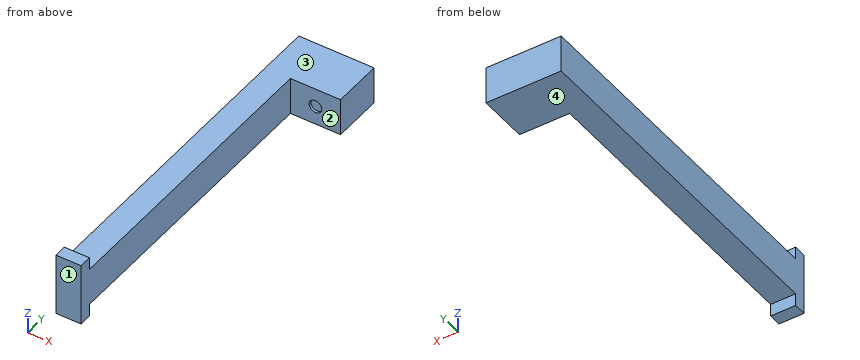
```python
from build123d import *

# Parameters (mm, degrees)
SKETCH2_W                = 30
SKETCH2_H                = 20
SKETCH2_W_2              = 10
SKETCH2_H_2              = 120
BOSS_EXTRUDE1_DEPTH      = 15
SKETCH3_W                = 10
SKETCH3_H                = 5
BOSS_EXTRUDE2_DEPTH      = 5
BOSS_EXTRUDE2_DEPTH_BACK = 20
SKETCH5_R                = 2.517277228
CUT_EXTRUDE1_DEPTH       = 1


with BuildPart() as part:
    # Sketch2 → Boss-Extrude1 (new body)
    with BuildSketch(Plane.XY):
        Rectangle(SKETCH2_W, SKETCH2_H)
        with Locations((-10, -70)):
            Rectangle(SKETCH2_W_2, SKETCH2_H_2)
    extrude(amount=BOSS_EXTRUDE1_DEPTH)

    # Sketch3 → Boss-Extrude2 (add, two sides)
    with BuildSketch(Plane.XY.offset(15)) as boss_extrude2_sk:
        with Locations((-10, -132.5)):
            Rectangle(SKETCH3_W, SKETCH3_H)
    extrude(amount=BOSS_EXTRUDE2_DEPTH)
    extrude(boss_extrude2_sk.sketch, amount=-BOSS_EXTRUDE2_DEPTH_BACK)

    # Sketch5 → Cut-Extrude1 (cut)
    with BuildSketch(Plane.XZ.offset(10)):
        with Locations((5, 7.5)):
            Circle(SKETCH5_R)
    extrude(amount=-CUT_EXTRUDE1_DEPTH, mode=Mode.SUBTRACT)


solid = part.part
```
Input: part model. Units: mm. Frame: model coordinates. Face numbers are marked on the shaded views. A direction names the side the tool comes from. Round coordinates to 2 decimals unless told otherwise and drop trailing zeros. Loops run counter-clockwise (first coordinate to the right, second up) from the corner with the lowest first, then second, coordinate; pieces in that order, holes last. Notation, with made-up numbers: (51.25, 63) -> (92.25, 63) arc R24 cw to (92.25, 84) -> close; hole circle Ø6 at (-4.75, 57). An arc over 180 degrees is marked (long way). One line per item, written item: value.
(1) Material intervals for line 1 (Z direction, x = 5, y = -9.45); line 2 (Z direction, x = 11.5, y = -7); line 3 (X direction, y = -11, z = 10), sorted ascending. Write a range as [from, to].
Geometry check:
line 1: [0, 4.98], [10.02, 15]
line 2: [0, 15]
line 3: [-15, -5]
(2) Set-up query: the marked faces 1, 2, 3 and 4. Return all of +Z, -Z, +X, -X, +Y, -Y with unobstructed straight access to the full face (end or side cutting, diameter ignored); none if empty.
Geometry check:
face 1: +Z, -Z, +X, -X, -Y
face 2: +Z, -Z, +X, -Y
face 3: +Z, +X, -X, +Y
face 4: -Z, +X, -X, +Y
(3) Section A-A (x = 5). Return the cut outline in (y, z), plus the area to 3 significant figures.
Geometry check:
outline: (-10, 0) -> (10, 0) -> (10, 15) -> (-10, 15) -> (-10, 10.02) -> (-9, 10.02) -> (-9, 4.98) -> (-10, 4.98) -> close
area: 295 mm2
(4) Pin query (flat end, axial travel): pin 1 (10 mm diameter, centred on y = -111.5, z = 2.5, fed in from +X); pin 2 (12 mm diameter, centred on x = 6, z = 8.5, fed in from -Y); pin 3 (2.5 mm diameter, centred on x = -10, z = 17, fed in from +Y). Return the tip coordinate at first contact, or that it passes through.
Geometry check:
pin 1: x = -5
pin 2: y = -10
pin 3: y = -130
(5) Section B-B (z = 7.5). Return the cut outline in (x, y), plus the area to 3 significant figures.
Geometry check:
outline: (-15, -135) -> (-5, -135) -> (-5, -10) -> (2.48, -10) -> (2.48, -9) -> (7.52, -9) -> (7.52, -10) -> (15, -10) -> (15, 10) -> (-15, 10) -> close
area: 1,840 mm2
(6) Section D-D (x = -11.75). Return the cut outline in (y, z), plus the area to 4 significant figures.
Geometry check:
outline: (-135, -5) -> (-130, -5) -> (-130, 0) -> (10, 0) -> (10, 15) -> (-130, 15) -> (-130, 20) -> (-135, 20) -> close
area: 2,225 mm2
(7) Section C-C (y = -27). Return the cut outline in (x, z).
Geometry check:
outline: (-15, 0) -> (-5, 0) -> (-5, 15) -> (-15, 15) -> close
